Model file for the job. Use its own axes, mm. A direction names the side the tool comes from. Give positions to 0.01 mm unless a question says otherwise; leave off trailing zeros. Order: outer loops, then holes, each group sorted by start corner. A loop starts at its lowest first (then second) coordinate and runs counter-clockwise, first axis right, second up. Notation, with made-up numbers: (16, 22.5) - (44, 22.5) arc R16 cw to (44, 50.5) - close; hole circle Ø4 at (81, -1). An arc over 180 degrees is marked (long way). Use CSV: the item, a comma, the result in double quotes. Start each with the question number.
(1) Tool access for faces 1 (the cylindrical face through (3.09, -5.07, 0.38)), 2 (the cylindrical face through (3.09, 26.72, 0.38)), 3 (the cylindrical face through (5.074, 3.451, 16.111)): list every direction of +Z, -Z, +X, -X, +Y, -Y with a clear straight run to the whole face (end or side of a thin tool).
(2) Band-saw the part on D-D, the plane z = -9. Give the cut face in (x, y), then the cut area to 3 significant figures.
(3) Probe L1, parallel to Y at x = 1, z = -6; L2, parallel to X at y = 27, z = 0.5; L3, parallel to Z at x = -7, y = 2. List the from-to ranges inside material, lowest first.
(4) Drop flat-ended pins along their axis: pin 1 Ø6 at (y, z) = (37, 3.5) entering from +X; pin 2 Ø12 at (y, z) = (14.5, 1) entering from +X; pin 3 Ø6 at (x, y) = (3, 34) entering from +Z; pin 4 Ø12 at (y, z) = (6, 2) entering from -X. Give the stop position or say it passes through.
(5) Band-saw the part on C-C, the plane x = 0. Give the cut face in (y, z).
(6) Band-saw the part on A-A, the plane z = 0. Give the cut face in (x, y).
(7) Band-saw the part on B-B, the plane y = 38.5. Give the cut face in (x, z), then the cut area to 3 significant figures.
from build123d import *

# Parameters (mm, degrees)
SKETCH2_R                = 16.891
BOSS_EXTRUDE1_DEPTH      = 7
BOSS_EXTRUDE2_DEPTH      = 40
BOSS_EXTRUDE2_DEPTH_BACK = 17
SKETCH3_R                = 0.703637869


with BuildPart() as part:
    # Sketch2 → Boss-Extrude1 (new body)
    with BuildSketch(Plane(origin=(0, 0, 0), x_dir=(1, 0, 0), z_dir=(0, 1, 0))):
        with Locations(Location((0, 0, 0), (0, 0, 270))):
            Circle(SKETCH2_R)
    extrude(amount=BOSS_EXTRUDE1_DEPTH)

    # Sketch3 → Boss-Extrude2 (add, two sides: drawn at the far end of the back side and taken through both)
    with BuildSketch(Plane(origin=(0, 7, 0), x_dir=(1, 0, 0), z_dir=(0, 1, 0)).offset(-BOSS_EXTRUDE2_DEPTH_BACK)):
        with Locations(Location((-2.5, 0, 0), (0, 0, 270))):
            Circle(SKETCH3_R)
        with Locations(Location((2.5, 0, 0), (0, 0, 270))):
            Circle(SKETCH3_R)
    extrude(amount=BOSS_EXTRUDE2_DEPTH + BOSS_EXTRUDE2_DEPTH_BACK)


solid = part.part
Answer block:
1,face 1,"-Y"
1,face 2,"+Y"
1,face 3,"+Y, -Y"
2,outline,"(-14.29, 0) - (14.29, 0) - (14.29, 7) - (-14.29, 7) - close"
2,area,"200 mm2"
3,L1,"y = 0 to 7"
3,L2,"x = -3 to -2, 2 to 3"
3,L3,"z = -15.37 to 15.37"
4,pin 1,"stops at x = 3"
4,pin 2,"stops at x = 3.2"
4,pin 3,"stops at z = 0.7"
4,pin 4,"stops at x = -16.89"
5,outline,"(0, -16.89) - (7, -16.89) - (7, 16.89) - (0, 16.89) - close"
6,outline,"(-16.89, 0) - (-3.2, 0) - (-3.2, -10) - (-1.8, -10) - (-1.8, 0) - (1.8, 0) - (1.8, -10) - (3.2, -10) - (3.2, 0) - (16.89, 0) - (16.89, 7) - (3.2, 7) - (3.2, 47) - (1.8, 47) - (1.8, 7) - (-1.8, 7) - (-1.8, 47) - (-3.2, 47) - (-3.2, 7) - (-16.89, 7) - close"
7,outline,"circle Ø1.41 at (-2.5, 0); circle Ø1.41 at (2.5, 0)"
7,area,"3.11 mm2"
